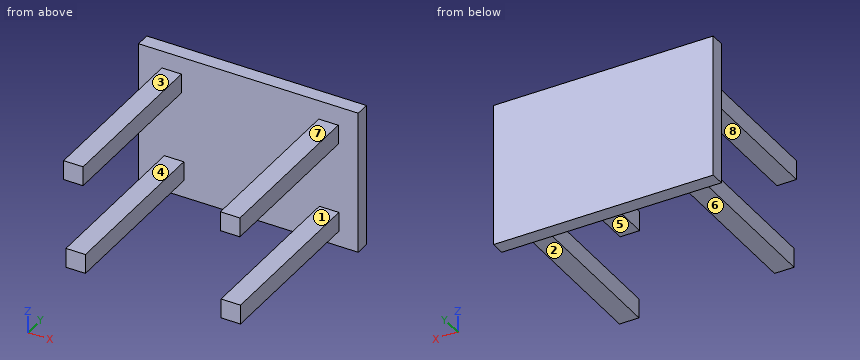
```python
from build123d import *

# Parameters (mm, degrees)
SKETCH1_W           = 155.20995072
SKETCH1_H           = 101.500935516
BOSS_EXTRUDE1_DEPTH = 10
SKETCH2_W           = 13.766131438
SKETCH2_H           = 13.766131439
SKETCH2_H_2         = 13.766131438
SKETCH2_W_2         = 13.766131439
BOSS_EXTRUDE2_DEPTH = 130


with BuildPart() as part:
    # Sketch1 → Boss-Extrude1 (new body)
    with BuildSketch(Plane(origin=(0, 0, 0), x_dir=(1, 0, 0), z_dir=(0, 1, 0))):
        Rectangle(SKETCH1_W, SKETCH1_H)
    extrude(amount=-BOSS_EXTRUDE1_DEPTH)

    # Sketch2 → Boss-Extrude2 (add)
    with BuildSketch(Plane(origin=(0, 0, 0), x_dir=(1, 0, 0), z_dir=(0, 1, 0))):
        with Locations((57.048171322, 33.010928537)):
            Rectangle(SKETCH2_W, SKETCH2_H)
        with Locations((-52.536052633, 31.886855475)):
            Rectangle(SKETCH2_W, SKETCH2_H_2)
        with Locations((-54.221701381, -31.605914017)):
            Rectangle(SKETCH2_W_2, SKETCH2_H_2)
        with Locations((56.609703773, -30.482148186)):
            Rectangle(SKETCH2_W, SKETCH2_H)
    extrude(amount=-BOSS_EXTRUDE2_DEPTH)


solid = part.part
```
The listing builds one solid part. Answer for the finished solid, in the listing's coordinates (mm). Face numbers are marked on the shaded views. A direction names the side the tool comes from. Round coordinates to 2 decimals unless told otherwise and drop trailing zeros. Loops run counter-clockwise (first coordinate to the right, second up) from the corner with the lowest first, then second, coordinate; pieces in that order, holes last. Notation, with made-up numbers: (32.25, 22) - (82.25, 22) arc R21 cw to (82.25, 49) - close; hole circle Ø3 at (33, 40.25). An arc over 180 degrees is marked (long way). Return JSON: item names as keys, results as strings. Group by question number.
1. The mould has two halves that part along Z. Classify the marked faces 5, 6, 7 and 8: pulls with the +Z half, pulls with the -Z half, needs draft (parallel to the pull), parting line crosses it, or undercut.
2. Each of these flat-tipped pins is pushed along its axis until it touches: P1, Ø7, axis at y = -78, z = 28.5, coming from the +X side; P2, Ø4, axis at x = 53.5, y = -63.5, coming from the +Z side; P3, Ø4, axis at y = -94.5, z = 30, coming from the -X side. Where does it stop, or does it pass through?
3. Which of the six approach directions +Z, -Z, +X, -X, +Y, -Y give full straight-line access (tool end or side, diameter ignored) to the marked faces 1, 2, 3 and 4?
4. The part is cut by section A-A on y = -53.5. Determine the outline of the cut face in (x, z), then the cut area to 3 significant figures.
5. Consider probe 1 along Y at (x, z) = (-5, -17.5); probe 2 along X at (y, z) = (-49.5, 35.5); probe 3 along Z at (x, y) = (60, -83.5). Determine where each line is inside the solid, lowest interval first.
6. The part is cut by section C-C on z = 28. Determine the outline of the cut face in (x, y), then the cut area to 3 significant figures.
7. The part is cut by section D-D on z = -16. Determine the outline of the cut face in (x, y).
8. The part is cut by section B-B on x = -55. Determine the outline of the cut face in (y, z), then the cut area to 3 significant figures.
Resolved:
{
 "1": {"face 5": "undercut", "face 6": "pulls with the -Z half", "face 7": "pulls with the +Z half", "face 8": "undercut"},
 "2": {"P1": "stops at x = 63.49", "P2": "stops at z = 37.37", "P3": "stops at x = -61.1"},
 "3": {"face 1": "+X, -Y", "face 2": "-Z, +X, -X, -Y", "face 3": "+Z, +X, -X, -Y", "face 4": "+X, -X, -Y"},
 "4": {"outline": "(-61.1, 24.72) - (-47.34, 24.72) - (-47.34, 38.49) - (-61.1, 38.49) - close; (-59.42, -38.77) - (-45.65, -38.77) - (-45.65, -25) - (-59.42, -25) - close; (49.73, 23.6) - (63.49, 23.6) - (63.49, 37.37) - (49.73, 37.37) - close; (50.17, -39.89) - (63.93, -39.89) - (63.93, -26.13) - (50.17, -26.13) - close", "area": "758 mm²"},
 "5": {"probe 1": "y = -10 to 0", "probe 2": "x = -61.1 to -47.34, 49.73 to 63.49", "probe 3": "z = -39.89 to -26.13, 23.6 to 37.37"},
 "6": {"outline": "(-77.6, -10) - (-61.1, -10) - (-61.1, -130) - (-47.34, -130) - (-47.34, -10) - (49.73, -10) - (49.73, -130) - (63.49, -130) - (63.49, -10) - (77.6, -10) - (77.6, 0) - (-77.6, 0) - close", "area": "4,860 mm²"},
 "7": {"outline": "(-77.6, -10) - (77.6, -10) - (77.6, 0) - (-77.6, 0) - close"},
 "8": {"outline": "(-130, -38.77) - (-10, -38.77) - (-10, -50.75) - (0, -50.75) - (0, 50.75) - (-10, 50.75) - (-10, 38.49) - (-130, 38.49) - (-130, 24.72) - (-10, 24.72) - (-10, -25) - (-130, -25) - close", "area": "4,320 mm²"}
}
